Input: part model. Units: mm. Frame: model coordinates. Face numbers are marked on the shaded views. Round coordinates to 2 decimals unless told otherwise and drop trailing zeros. Loops run counter-clockwise (first coordinate to the right, second up) from the corner with the lowest first, then second, coordinate; pieces in that order, holes last. Notation, with made-up numbers: (2, 12.25) - (55, 12.25) arc R26 ccw to (55, 42.25) - close; hole circle Ø5 at (-22.5, -30). An arc over 180 degrees is marked (long way). One line per question, with ' | ' between items. Start each with the question number.
Item 1: Draft query along X for the marked faces 1, 2 and 3. Return one class per face: pulls with the +X half, pulls with the -X half, needs draft (parallel to the pull), parting line crosses it, or undercut.
Item 2: Section C-C, the plane z = -37.5. Return loops of the section in (x, y).
Item 3: Section A-A, the plane y = 5.25. Return loops of the section in (x, z).
Item 4: First-contact query: pin 1 (8 mm diameter, centred on x = -38, y = 10, fed in from +Z); pin 2 (4 mm diameter, centred on y = 2, z = -35, fed in from +X); pin 3 (6 mm diameter, centred on y = 2, z = 14, fed in from -X). Flat tips, straight axial feed; report the tip coordinate or a pass-through.
Item 5: Section B-B, the plane x = 54. Return loops of the section in (y, z).
Item 6: Material intervals for line 1 along Z through (x, y) = (-23, 11); line 2 along Z through (x, y) = (-12, 2.25); line 3 along Y through (x, z) = (-33, -16), sorted ascending.
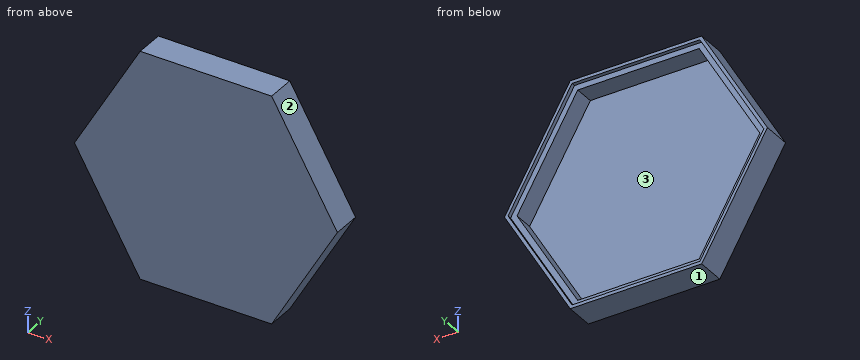
```python
from build123d import *

# Parameters (mm, degrees)
BOSS_EXTRUDE1_DEPTH = 2.4
BOSS_EXTRUDE2_DEPTH = 10
BOSS_EXTRUDE3_DEPTH = 12


with BuildPart() as part:
    # Sketch1 → Boss-Extrude1 (new body)
    with BuildSketch(Plane(origin=(0, 0, 0), x_dir=(1, 0, 0), z_dir=(0, 1, 0))):
        Polygon((66.395280957, 0), (33.197640478, 57.5), (-33.197640478, 57.5), (-66.395280957, 0), (-33.197640478, -57.5), (33.197640478, -57.5), align=None)
    extrude(amount=-BOSS_EXTRUDE1_DEPTH)

    # Sketch1<3> → Boss-Extrude2 (add)
    with BuildSketch(Plane(origin=(0, 0, 0), x_dir=(1, 0, 0), z_dir=(0, 1, 0))):
        Polygon((32.273880048, -55.9), (64.547760095, 0), (32.273880048, 55.9), (-32.273880048, 55.9), (-64.547760095, 0), (-32.273880048, -55.9), align=None)
        Polygon((30.657299294, 53.1), (-30.657299294, 53.1), (-61.314598588, 0), (-30.657299294, -53.1), (30.657299294, -53.1), (61.314598588, 0), align=None, mode=Mode.SUBTRACT)
    extrude(amount=BOSS_EXTRUDE2_DEPTH)

    # Sketch1<4> → Boss-Extrude3 (add)
    with BuildSketch(Plane(origin=(0, 0, 0), x_dir=(1, 0, 0), z_dir=(0, 1, 0))):
        Polygon((-33.197640478, -57.5), (33.197640478, -57.5), (66.395280957, 0), (33.197640478, 57.5), (-33.197640478, 57.5), (-66.395280957, 0), align=None)
        Polygon((64.547760095, 0), (32.273880048, 55.9), (-32.273880048, 55.9), (-64.547760095, 0), (-32.273880048, -55.9), (32.273880048, -55.9), align=None, mode=Mode.SUBTRACT)
    extrude(amount=BOSS_EXTRUDE3_DEPTH)


solid = part.part
```
Return value:
1) face 1: needs draft | face 2: pulls with the +X half | face 3: undercut
2) outline: (-44.74, -2.4) - (44.74, -2.4) - (44.74, 12) - (42.9, 12) - (42.9, 10) - (39.66, 10) - (39.66, 0) - (-39.66, 0) - (-39.66, 10) - (-42.9, 10) - (-42.9, 12) - (-44.74, 12) - close
3) outline: (-66.4, 0) - (-33.2, -57.5) - (33.2, -57.5) - (66.4, 0) - (33.2, 57.5) - (-33.2, 57.5) - close; hole (-61.31, 0) - (-30.66, -53.1) - (30.66, -53.1) - (61.31, 0) - (30.66, 53.1) - (-30.66, 53.1) - close
4) pin 1: z = 56.11 | pin 2: x = 47.34 | pin 3: x = -60.04
5) outline: (-2.4, -21.47) - (12, -21.47) - (12, -18.27) - (10, -18.27) - (10, -12.67) - (0, -12.67) - (0, 12.67) - (10, 12.67) - (10, 18.27) - (12, 18.27) - (12, 21.47) - (-2.4, 21.47) - close
6) line 1: -57.5 to -55.9, 55.9 to 57.5 | line 2: -57.5 to -53.1, 53.1 to 57.5 | line 3: -2.4 to 0
